Verification items for the finished model (mm, model axes). Face numbers are marked on the shaded views. A direction names the side the tool comes from. Coordinates: 2 decimals unless noted, no trailing zeros. Write each loop counter-clockwise with the first axis right and the second up, starting at its lowest first coordinate (ties: lowest second). Pieces come first, ordered by that corner, then holes. Notation, with made-up numbers: (46, 66.5) -> (103, 66.5) arc R28 cw to (103, 92.5) -> close; hole circle Ø11 at (34, 25.25). An arc over 180 degrees is marked (long way). Write item = value, one per line. Start each with the question number.
(1) Section check D-D (y = -9.5). Record the cut outline in (x, z).
(2) Mould release check, pull along Z, two halves, no side actions. Record for the marked faces 1, 2 and 3: released by +Z, released by -Z, zero draft, split by the parting line, or undercut.
(3) Section check B-B (z = -25.4). Record the cut outline in (x, y).
(4) Section check C-C (x = 89). Record the cut outline in (y, z).
(5) Section check A-A (x = -101.6). Record the cut outline in (y, z), plus the area to 3 significant figures.
(6) Material ranges on probe 1 along Y at (x, z) = (231.5, -36.5); probe 2 along Y at (x, z) = (155.5, -96); probe 3 along Z at (x, y) = (27, -83), recorded low to high. Write a range as [from, to].
(7) Gauge pin test, flat ends, axial feed: pin 1 Ø4 at (x, z) = (146.5, 116) entering from +Y; pin 2 Ø6 at (y, z) = (-116.5, -60.5) entering from +X; pin 3 Ø5 at (y, z) = (189.5, -139.5) entering from +X. Record the tip position at first contact, or that the pin passes through.
(8) Set-up check for the marked faces 4, 5 and 6: record each of +Z, -Z, +X, -X, +Y, -Y from which the full face is reachable in a straight line by a thin tool's end or side.
```python
from build123d import *

# Parameters (mm, degrees)
BOSS_EXTRUDE3_DEPTH  = 38.1
BOSS_EXTRUDE4_START  = -38.1
SKETCH2_R            = 101.6
SKETCH2_R_2          = 63.5
BOSS_EXTRUDE4_DEPTH  = 38.1
BOSS_EXTRUDE5_START  = -127
BOSS_EXTRUDE5_DEPTH  = 127
BOSS_EXTRUDE7_START  = 88.9
BOSS_EXTRUDE7_DEPTH  = 88.9
BOSS_EXTRUDE8_DEPTH  = 38.1
SKETCH9_R            = 190.5
BOSS_EXTRUDE9_DEPTH  = 50.8
SKETCH15_R           = 127
BOSS_EXTRUDE10_DEPTH = 152.4
SKETCH16_R           = 12.7
BOSS_EXTRUDE11_DEPTH = 50.8
SKETCH17_R           = 63.5
CUT_EXTRUDE1_DEPTH   = 25.4
BOSS_EXTRUDE12_DEPTH = 50.8


with BuildPart() as part:
    # Sketch1 → Boss-Extrude3 (new body)
    with BuildSketch(Plane.XY):
        with BuildLine():
            ThreePointArc((0, 175.976362049), (-66.179327011, 80.750651629), (-178.502675689, 109.579536282))
            Line((-178.502675689, 109.579536282), (-48.064172306, -41.498016104))
            ThreePointArc((-48.064172306, -41.498016104), (-31.75, 54.99261314), (59.970422306, 20.875786176))
            Line((59.970422306, 20.875786176), (-5.647324311, 209.377619931))
            ThreePointArc((-5.647324311, 209.377619931), (-1.421779188, 192.914014631), (0, 175.976362049))
        make_face()
    extrude(amount=BOSS_EXTRUDE3_DEPTH)

    # Sketch2 → Boss-Extrude4 (add)
    with BuildSketch(Plane.XY.offset(38.1).offset(BOSS_EXTRUDE4_START)):
        with Locations((-101.6, 175.976362049)):
            Circle(SKETCH2_R)
        Circle(SKETCH2_R_2)
    extrude(amount=BOSS_EXTRUDE4_DEPTH)

    # Sketch3 → Boss-Extrude5 (add)
    with BuildSketch(Plane.XY.offset(38.1).offset(BOSS_EXTRUDE5_START)):
        with BuildLine():
            Line((-48.064172306, -41.498016104), (-48.064172306, -168.498016104))
            Line((-48.064172306, -168.498016104), (205.935827694, -168.498016104))
            Line((205.935827694, -168.498016104), (205.935827694, -92.298016104))
            Line((205.935827694, -92.298016104), (59.970422306, 20.875786176))
            ThreePointArc((59.970422306, 20.875786176), (31.75, -54.99261314), (-48.064172306, -41.498016104))
        make_face()
    extrude(amount=BOSS_EXTRUDE5_DEPTH)

    # Sketch4 → Boss-Extrude7 (add)
    with BuildSketch(Plane(origin=(0, 0, 0), x_dir=(-1, 0, 0), z_dir=(0, 0, -1)).offset(BOSS_EXTRUDE7_START)):
        with BuildLine():
            Line((-60.014697878, 20.748157474), (-18.263261234, 140.689049326))
            Line((-18.263261234, 140.689049326), (134.985164693, 59.176328053))
            Line((134.985164693, 59.176328053), (51.773850531, -36.765723184))
            ThreePointArc((51.773850531, -36.765723184), (-29.050636969, -56.465126332), (-60.014697878, 20.748157474))
        make_face()
    extrude(amount=-BOSS_EXTRUDE7_DEPTH)

    # Sketch11 → Boss-Extrude8 (add)
    with BuildSketch(Plane(origin=(0, 0, -88.9), x_dir=(-1, 0, 0), z_dir=(0, 0, -1))):
        with BuildLine():
            Line((13.737038838, 226.313954509), (-18.263261234, 140.689049326))
            Line((-18.263261234, 140.689049326), (134.985164693, 59.176328053))
            Line((134.985164693, 59.176328053), (189.462961162, 125.638769589))
            ThreePointArc((189.462961162, 125.638769589), (151.93759246, 263.839323211), (13.737038838, 226.313954509))
        make_face()
    extrude(amount=-BOSS_EXTRUDE8_DEPTH)

    # Sketch9 → Boss-Extrude9 (add)
    with BuildSketch(Plane(origin=(0, -168.498016104, 0), x_dir=(-1, 0, 0), z_dir=(0, -1, 0))):
        with Locations(Location((-78.935827694, 25.4, 0), (0, 0, 90))):
            Circle(SKETCH9_R)
    extrude(amount=BOSS_EXTRUDE9_DEPTH)

    # Sketch15 → Boss-Extrude10 (add)
    with BuildSketch(Plane.XZ.offset(219.298016104)):
        with Locations(Location((78.692071522, -25.762296975, 0), (0, 0, 90))):
            Circle(SKETCH15_R)
    extrude(amount=BOSS_EXTRUDE10_DEPTH)

    # Sketch16 → Boss-Extrude11 (add)
    with BuildSketch(Plane.XY.offset(-50.8)):
        with Locations(Location((-101.6, 175.976362049, 0), (0, 0, 180))):
            Circle(SKETCH16_R)
    extrude(amount=BOSS_EXTRUDE11_DEPTH)

    # Sketch17 → Cut-Extrude1 (cut)
    with BuildSketch(Plane.XZ.offset(371.698016104)):
        with Locations(Location((78.692071522, -25.762296975, 0), (0, 0, 270))):
            Circle(SKETCH17_R)
    extrude(amount=-CUT_EXTRUDE1_DEPTH, mode=Mode.SUBTRACT)

    # Sketch19 → Boss-Extrude12 (add)
    with BuildSketch(Plane.XY.offset(38.1)):
        Polygon((-24.564880981, 119.003650496), (-75.267213011, 207.048147921), (-141.300586079, 169.021398898), (-90.598254049, 80.976901474), align=None)
    boss_extrude12 = extrude(amount=BOSS_EXTRUDE12_DEPTH)

    # Mirror1: Boss-Extrude12 across plane
    add(boss_extrude12.mirror(Plane(origin=(0, 0, -25.4), x_dir=(1, 0, 0), z_dir=(0, 0, -1))))


solid = part.part
```
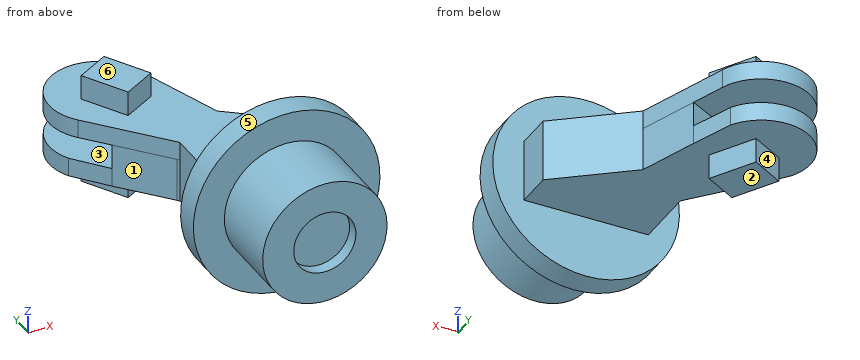
Response:
q1.outline = (-75.69, 0) -> (-75.42, 0) -> (-75.42, -88.9) -> (99.15, -88.9) -> (99.15, 38.1) -> (-75.69, 38.1) -> close
q2.face_1 = zero draft
q2.face_2 = released by -Z
q2.face_3 = undercut
q3.outline = (-134.99, 59.18) -> (-51.77, -36.77) arc R63.5 ccw to (-48.06, -41.5) -> (-48.06, -168.5) -> (-111.56, -168.5) -> (-111.56, -219.3) -> (-48.31, -219.3) -> (-48.31, -371.7) -> (15.19, -371.7) -> (15.19, -346.3) -> (142.19, -346.3) -> (142.19, -371.7) -> (205.69, -371.7) -> (205.69, -219.3) -> (269.44, -219.3) -> (269.44, -168.5) -> (205.94, -168.5) -> (205.94, -92.3) -> (59.97, 20.88) arc R63.5 cw to (60.01, 20.75) -> (18.26, 140.69) -> close; circle Ø25.4 at (-101.6, 175.98)
q4.outline = (-371.7, -152.34) -> (-219.3, -152.34) -> (-219.3, -215.63) -> (-168.5, -215.63) -> (-168.5, -88.9) -> (-1.63, -88.9) -> (-1.63, 38.1) -> (-168.5, 38.1) -> (-168.5, 164.83) -> (-219.3, 164.83) -> (-219.3, 100.82) -> (-371.7, 100.82) -> (-371.7, 36.9) -> (-346.3, 36.9) -> (-346.3, -88.42) -> (-371.7, -88.42) -> close
q5.outline = (-219.3, -86.2) -> (-168.5, -86.2) -> (-168.5, 35.4) -> (-219.3, 35.4) -> close; (20.51, 0) -> (20.68, 0) -> (20.68, -88.9) -> (100.08, -88.9) -> (100.08, -139.7) -> (191.88, -139.7) -> (191.88, -88.9) -> (277.24, -88.9) -> (277.24, -50.8) -> (188.68, -50.8) -> (188.68, 0) -> (277.58, 0) -> (277.58, 38.1) -> (191.88, 38.1) -> (191.88, 88.9) -> (100.08, 88.9) -> (100.08, 38.1) -> (20.51, 38.1) -> close; hole (76.93, -50.8) -> (163.28, -50.8) -> (163.28, 0) -> (76.93, 0) -> close
q5.area = 39,200 mm2
q6.probe_1 = [-219.3, -168.5]
q6.probe_2 = [-371.7, -168.5]
q6.probe_3 = [-88.9, 38.1]
q7.pin_1 = -168.5
q7.pin_2 = 205.94
q7.pin_3 = -63.72
q8.face_4 = -Z, -X, +Y
q8.face_5 = -Y
q8.face_6 = +Z, +X, -X, +Y
